Geometry check sheet. Reference: the model listing, model coordinates, mm. A direction names the side the tool comes from. Give positions to 0.01 mm unless a question says otherwise; leave off trailing zeros. Order: outer loops, then holes, each group sorted by start corner. A loop starts at its lowest first (then second) coordinate and runs counter-clockwise, first axis right, second up. Notation, with made-up numbers: (-17.75, -6) - (-6.75, -6) arc R26 ccw to (-6.75, 31) - close; hole circle Ø9 at (-25.75, 79.5). An arc over 180 degrees is marked (long way). Put each result on its own line as item: value. Start each with the question number.
```python
from build123d import *

# Parameters (mm, degrees)
BOSS_EXTRUDE1_DEPTH = 9.2
SKETCH2_W           = 0.75
SKETCH2_H           = 17.4
SKETCH3_R           = 1.5
BOSS_EXTRUDE2_DEPTH = 4.8
SKETCH4_R           = 0.25
BOSS_EXTRUDE3_DEPTH = 3.35
SKETCH5_R           = 1.35
CUT_EXTRUDE1_DEPTH  = 10.2


with BuildPart() as part:
    # Sketch1 → Boss-Extrude1 (new body)
    with BuildSketch(Plane(origin=(0, 0, 0), x_dir=(1, 0, 0), z_dir=(0, 1, 0))):
        with BuildLine():
            Line((-32, 17.5), (32, 17.5))
            ThreePointArc((32, 17.5), (49.5, 0), (32, -17.5))
            Line((32, -17.5), (-32, -17.5))
            ThreePointArc((-32, -17.5), (-49.5, 0), (-32, 17.5))
        make_face()
    extrude(amount=-BOSS_EXTRUDE1_DEPTH)

    # Sketch2 → Revolve1 (revolve)
    with BuildSketch(Plane(origin=(9.5, 0, 0), x_dir=(0, 0, -1), z_dir=(1, 0, 0))):
        with Locations((0.375, 8.7)):
            Rectangle(SKETCH2_W, SKETCH2_H)
        Polygon((1, 0), (2.947531596, 0), (2.5, 6.4), (2, 6.4), (2, 11.2), (1, 11.2), align=None)
    revolve(axis=Axis((9.5, 0, 0), (0, 1, 0)))

    # Sketch3 → Boss-Extrude2 (add)
    with BuildSketch(Plane(origin=(0, 0, 0), x_dir=(1, 0, 0), z_dir=(0, 1, 0))):
        with Locations((0, -12)):
            Circle(SKETCH3_R)
        with Locations((30, 9)):
            Circle(SKETCH3_R)
        with Locations((-30, 9)):
            Circle(SKETCH3_R)
    extrude(amount=BOSS_EXTRUDE2_DEPTH)

    # Sketch4 → Boss-Extrude3 (add)
    with BuildSketch(Plane(origin=(0, 0, 0), x_dir=(1, 0, 0), z_dir=(0, 1, 0))):
        with Locations((-19.32, 11.425)):
            Circle(SKETCH4_R)
        with Locations((-11.62, 11.425)):
            Circle(SKETCH4_R)
        with Locations((-11.62, -11.425)):
            Circle(SKETCH4_R)
        with Locations((-19.32, -11.425)):
            Circle(SKETCH4_R)
        with Locations((19.32, -11.425)):
            Circle(SKETCH4_R)
        with Locations((11.62, -11.425)):
            Circle(SKETCH4_R)
        with Locations((11.62, 11.425)):
            Circle(SKETCH4_R)
        with Locations((19.32, 11.425)):
            Circle(SKETCH4_R)
    extrude(amount=BOSS_EXTRUDE3_DEPTH)

    # Sketch5 → Cut-Extrude1 (cut, through all)
    with BuildSketch(Plane(origin=(0, 0, 0), x_dir=(1, 0, 0), z_dir=(0, 1, 0))):
        with Locations((0, 15.1)):
            Circle(SKETCH5_R)
        with Locations((0, -15.1)):
            Circle(SKETCH5_R)
    extrude(amount=-CUT_EXTRUDE1_DEPTH, mode=Mode.SUBTRACT)


solid = part.part
```
Item 1: Release check for a two-part mould opening along X. For faces 1 (the face through (7.517, 8.834, 0.26)), 2 (the face through (-0.176, -4.536, -16.439)), 3 (the face through (10.4, 11.2, -0.9)) record: +X half, -X half, draft (parallel to the pull), parting line (faces both ways), or undercut.
Item 2: Gauge pin test, flat ends, axial feed: pin 1 Ø5 at (y, z) = (0, -9) entering from +X; pin 2 Ø8 at (x, z) = (29.5, 1.5) entering from +Y; pin 3 Ø0.6 at (x, z) = (-11.5, -11.5) entering from +Y; pin 4 Ø3 at (x, z) = (0, -15.1) entering from -Y. Record the tip position at first contact, or that the pin passes through.
Item 3: Thickness scan on line 1 along Z through (x, y) = (0, -6.5); line 2 along Z through (x, y) = (9.5, 2.5); line 3 along X through (y, z) = (5, 0). Record the ranges inside material, lowest first.
Item 4: Cross-section at C-C (y = -7). Enter the section's corners in (x, z).
Item 5: Cross-section at D-D (x = -25). Enter the section's corners in (y, z).
Item 6: Set-up check for faces 4 (the face through (0, 4.8, 12)), 5 (the face through (-31.5, 2.37, -9.07)): record each of +Z, -Z, +X, -X, +Y, -Y from which the full face is reachable in a straight line by a thin tool's end or side.
Item 7: Cross-section at A-A (y = 8.5). Enter the section's corners in (x, z).
Item 8: Cross-section at B-B (z = -9). Enter the section's corners in (x, y), and give its area (3 significant figures).
Recorded:
1. face 1: parting line
1. face 2: undercut
1. face 3: draft
2. pin 1: stops at x = 48.25
2. pin 2: stops at y = 0
2. pin 3: stops at y = 3.35
2. pin 4: stops at y = -9.2
3. line 1: z = -17.5 to -16.45, -13.75 to 13.75, 16.45 to 17.5
3. line 2: z = -2.77 to -1, -0.75 to 0.75, 1 to 2.77
3. line 3: x = 6.9 to 8.5, 8.75 to 10.25, 10.5 to 12.1
4. outline: (-32, -17.5) - (32, -17.5) arc R17.5 ccw to (32, 17.5) - (-32, 17.5) arc R17.5 ccw to start; hole circle Ø2.7 at (0, -15.1); hole circle Ø2.7 at (0, 15.1)
5. outline: (-9.2, -17.5) - (0, -17.5) - (0, 17.5) - (-9.2, 17.5) - close
6. face 4: +Z, -Z, +X, -X, +Y
6. face 5: +Y
7. outline: circle Ø4 at (9.5, 0); circle Ø1.5 at (9.5, 0); hole circle Ø2 at (9.5, 0)
8. outline: (-47.01, -9.2) - (47.01, -9.2) - (47.01, 0) - (31.5, 0) - (31.5, 4.8) - (28.5, 4.8) - (28.5, 0) - (-28.5, 0) - (-28.5, 4.8) - (-31.5, 4.8) - (-31.5, 0) - (-47.01, 0) - close
8. area: 894 mm^2
